Autodesk Inventor part; units mm, degrees
ref_plane "YZ Plane" through (0, 0, 0) normal (1, 0, 0) x (0, 1, 0)
ref_plane "XZ Plane" through (0, 0, 0) normal (0, 1, 0) x (-1, 0, 0)
ref_plane "XY Plane" through (0, 0, 0) normal (0, 0, 1) x (1, 0, 0)
sketch "Sketch1" plane through (0, 0, 0) normal (0, 1, 0) x (-1, 0, 0)
  line L0 (0, 0) -> (90, 0)
  line L1 (90, 0) -> (90, -90)
  line L2 (90, -90) -> (0, -90)
  line L3 (0, -90) -> (0, 0)
  dimension "d0" = 90
  dimension "d1" = 90
extrude "Extrusion1" add sketch "Sketch1" along normal blind 5
sketch "Sketch2" plane through (0, 5, 0) normal (0, 1, 0) x (1, 0, 0)
  line L0 (-5, 5) -> (-85, 5)
  line L1 (-85, 5) -> (-85, 85)
  line L2 (-85, 85) -> (-5, 85)
  line L3 (-5, 85) -> (-5, 5)
  line L4 (0, 0) -> (0, 90)
  line L5 (-90, 0) -> (0, 0)
  line L6 (-10, 10) -> (-80, 10)
  line L7 (-80, 10) -> (-80, 80)
  line L8 (-80, 80) -> (-10, 80)
  line L9 (-10, 80) -> (-10, 10)
  dimension "d4" = 5
  dimension "d5" = 5
  dimension "d6" = 80
  dimension "d7" = 80
  dimension "d8" = 5
  dimension "d9" = 5
  dimension "d10" = 70
  dimension "d11" = 70
extrude "Extrusion2" add sketch "Sketch2" along normal blind 10
sketch "Sketch3" plane through (0, 5, 0) normal (0, 1, 0) x (1, 0, 0)
  circle A0 centre (-45, 45) radius 3.5
  line L0 (0, 0) -> (0, 90)
  line L1 (0, 90) -> (-90, 90)
  dimension "d14" = 45
  dimension "d15" = 45
  dimension "d16" = 7
extrude "Extrusion3" cut sketch "Sketch3" against normal blind 10
properties part number "BlackBoxTopFall2019"
Work out the finished part from the listing and answer in its coordinate system (mm). A direction names the side the tool comes from. Round coordinates to 2 decimals unless told otherwise and drop trailing zeros. Order: outer loops, then holes, each group sorted by start corner. A loop starts at its lowest first (then second) coordinate and runs counter-clockwise, first axis right, second up. Notation, with made-up numbers: M 55.25,39.5 L 69.25,39.5 A18 cw 69.25,65.5 Z; hole C -36.75,-13.75 d5. An arc over 180 degrees is marked long. Put each result on its own line as item: value. Start each with the question number.
Q1. Flat-ended cylindrical pins translate along their axes: pin 1 (4 mm diameter, centred on y = 10.5, z = -51.5, fed in from -X); pin 2 (5 mm diameter, centred on x = -42.5, y = 11, fed in from +Z); pin 3 (5 mm diameter, centred on x = -50.5, y = 10.5, fed in from -Z). Find the tip coordinate at first contact, or state that the pin passes through.
Q2. A tool of negligible diameter and unlimited length cuts with its end or side. For faces 5 (the flat face through (-85, 10, -44)), 6 (the flat face through (-44, 10, -5)), 7 (the flat face through (-10, 10, -45)), from which of +Z, -Z, +X, -X, +Y, -Y can it reach the whole face along a straight path? Write none if from no direction.
Q3. Section C-C, the plane z = -45 is taken. Write down the section's boundary in (x, y), and give its area (3 significant figures).
Q4. For a pull along Z with two mould halves and no side action, classify faces 1 (the flat face through (-44, 2, 0)), 2 (the flat face through (-46, 2, -90)), 3 (the flat face through (-81, 15, -45)), 4 (the flat face through (-80, 10, -45)) as pulls with the +Z half, pulls with the -Z half, needs draft (parallel to the pull), parting line crosses it, or undercut.
Q5. Section B-B, the plane y = 8.5 is taken. Write down the section's boundary in (x, z), and give its area (3 significant figures).
Q6. Section A-A, the plane x = -45 is taken. Write down the section's boundary in (y, z).
Q7. Straight lines are drawn through the part: L1, parallel to Z at x = -45, y = 2.75; L2, parallel to X at y = 12.5, z = -45. For each, find the intervals that lie inside material, in ascending order. Write a range as [from, to].
Q8. Section D-D, the plane z = -8 is taken. Write down the section's boundary in (x, y).
Findings below:
1. pin 1: stops at x = -85
1. pin 2: stops at z = -5
1. pin 3: stops at z = -85
2. face 5: +Z, -Z, -X, +Y
2. face 6: +Z, +X, -X, +Y
2. face 7: +Y
3. outline: M -90,0 L -48.5,0 L -48.5,5 L -80,5 L -80,15 L -85,15 L -85,5 L -90,5 Z; M -41.5,0 L 0,0 L 0,5 L -5,5 L -5,15 L -10,15 L -10,5 L -41.5,5 Z
3. area: 515 mm^2
4. face 1: pulls with the +Z half
4. face 2: pulls with the -Z half
4. face 3: needs draft
4. face 4: undercut
5. outline: M -85,-85 L -5,-85 L -5,-5 L -85,-5 Z; hole M -80,-80 L -10,-80 L -10,-10 L -80,-10 Z
5. area: 1,500 mm^2
6. outline: M 0,-90 L 5,-90 L 5,-85 L 15,-85 L 15,-80 L 5,-80 L 5,-48.5 L 0,-48.5 Z; M 0,-41.5 L 5,-41.5 L 5,-10 L 15,-10 L 15,-5 L 5,-5 L 5,0 L 0,0 Z
7. L1: z = [-90, -48.5], [-41.5, 0]
7. L2: x = [-85, -80], [-10, -5]
8. outline: M -90,0 L 0,0 L 0,5 L -5,5 L -5,15 L -85,15 L -85,5 L -90,5 Z
